from build123d import *

# Parameters (mm, degrees)
F1_DEPTH = 2
F2_DEPTH = 100
F4_DEPTH = 28.001


with BuildPart() as f1:
    # F0 (on Top) → F1 (new body)
    with BuildSketch(Plane.XY):
        with BuildLine():
            ThreePointArc((23.5, 0), (19.9852813742, 8.4852813742), (11.5, 12))
            Line((11.5, 12), (-4.2888974491, 12))
            ThreePointArc((-4.2888974491, 12), (0.6851433252, 6.8936407031), (2.5, 0))
            ThreePointArc((2.5, 0), (0.6851433252, -6.8936407031), (-4.2888974491, -12))
            Line((-4.2888974491, -12), (11.5, -12))
            ThreePointArc((11.5, -12), (19.9852813742, -8.4852813742), (23.5, 0))
        make_face()
        with BuildLine():
            ThreePointArc((2.5, 0), (0.6851433252, 6.8936407031), (-4.2888974491, 12))
            Line((-4.2888974491, 12), (-11.5, 12))
            ThreePointArc((-11.5, 12), (-19.9852813742, 8.4852813742), (-23.5, 0))
            ThreePointArc((-23.5, 0), (-19.9852813742, -8.4852813742), (-11.5, -12))
            Line((-11.5, -12), (-4.2888974491, -12))
            ThreePointArc((-4.2888974491, -12), (0.6851433252, -6.8936407031), (2.5, 0))
        make_face()
        with BuildLine():
            Line((-4.2888974491, 12), (11.5, 12))
            ThreePointArc((11.5, 12), (19.9852813742, 8.4852813742), (23.5, 0))
            ThreePointArc((23.5, 0), (19.9852813742, -8.4852813742), (11.5, -12))
            Line((11.5, -12), (-4.2888974491, -12))
            ThreePointArc((-4.2888974491, -12), (-7.7583426132, -13.4907375632), (-11.5, -14))
            Line((-11.5, -14), (11.5, -14))
            ThreePointArc((11.5, -14), (21.3994949366, -9.8994949366), (25.5, 0))
            ThreePointArc((25.5, 0), (21.3994949366, 9.8994949366), (11.5, 14))
            Line((11.5, 14), (-11.5, 14))
            ThreePointArc((-11.5, 14), (-7.7583426132, 13.4907375632), (-4.2888974491, 12))
        make_face()
        with BuildLine():
            Line((-11.5, 12), (-4.2888974491, 12))
            ThreePointArc((-4.2888974491, 12), (-7.7583426132, 13.4907375632), (-11.5, 14))
            ThreePointArc((-11.5, 14), (-25.5, 0), (-11.5, -14))
            ThreePointArc((-11.5, -14), (-7.7583426132, -13.4907375632), (-4.2888974491, -12))
            Line((-4.2888974491, -12), (-11.5, -12))
            ThreePointArc((-11.5, -12), (-19.9852813742, -8.4852813742), (-23.5, 0))
            ThreePointArc((-23.5, 0), (-19.9852813742, 8.4852813742), (-11.5, 12))
        make_face()
    extrude(amount=F1_DEPTH)

    # F0 (on Top) → F2 (join)
    with BuildSketch(Plane.XY):
        with BuildLine():
            Line((-4.2888974491, 12), (11.5, 12))
            ThreePointArc((11.5, 12), (19.9852813742, 8.4852813742), (23.5, 0))
            ThreePointArc((23.5, 0), (19.9852813742, -8.4852813742), (11.5, -12))
            Line((11.5, -12), (-4.2888974491, -12))
            ThreePointArc((-4.2888974491, -12), (-7.7583426132, -13.4907375632), (-11.5, -14))
            Line((-11.5, -14), (11.5, -14))
            ThreePointArc((11.5, -14), (21.3994949366, -9.8994949366), (25.5, 0))
            ThreePointArc((25.5, 0), (21.3994949366, 9.8994949366), (11.5, 14))
            Line((11.5, 14), (-11.5, 14))
            ThreePointArc((-11.5, 14), (-7.7583426132, 13.4907375632), (-4.2888974491, 12))
        make_face()
        with BuildLine():
            Line((-11.5, 12), (-4.2888974491, 12))
            ThreePointArc((-4.2888974491, 12), (-7.7583426132, 13.4907375632), (-11.5, 14))
            ThreePointArc((-11.5, 14), (-25.5, 0), (-11.5, -14))
            ThreePointArc((-11.5, -14), (-7.7583426132, -13.4907375632), (-4.2888974491, -12))
            Line((-4.2888974491, -12), (-11.5, -12))
            ThreePointArc((-11.5, -12), (-19.9852813742, -8.4852813742), (-23.5, 0))
            ThreePointArc((-23.5, 0), (-19.9852813742, 8.4852813742), (-11.5, 12))
        make_face()
    extrude(amount=F2_DEPTH)

    # F3 (on face) → F4 (cut, through all)
    with BuildSketch(Plane(origin=(0, 14, 0), x_dir=(-1, 0, 0), z_dir=(0, 1, 0))):
        Polygon((-30, 127.5684932653), (-30, 100), (30, 80), (30, 127.5684932653), align=None)
    extrude(amount=-F4_DEPTH, mode=Mode.SUBTRACT)


solid = f1.part
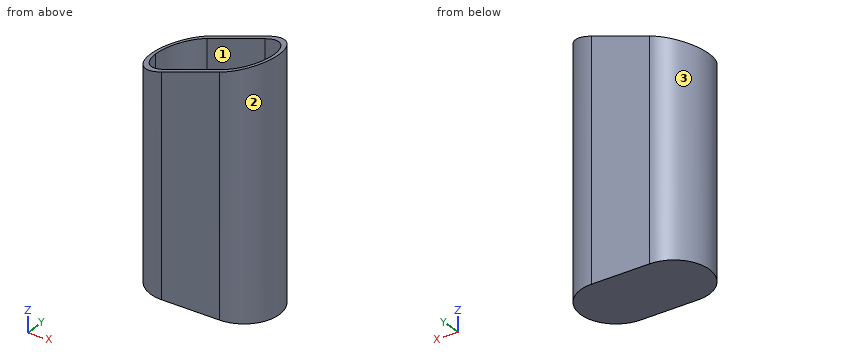
Input: part model. Units: mm. Frame: model coordinates. Face numbers are marked on the shaded views. Give positions to 0.01 mm unless a question says otherwise; leave off trailing zeros. Order: outer loops, then holes, each group sorted by start corner. A loop starts at its lowest first (then second) coordinate and runs counter-clockwise, first axis right, second up. Notation, with made-up numbers: (29, 78.5) - (76, 78.5) arc R11 ccw to (76, 94.5) - close; hole circle Ø9 at (14.5, 33.25). An arc over 180 degrees is marked (long way). Answer as a JSON object with one key per item and string values. Group by question number.
Q1. Cut plane C-C, the plane x = 20. Output: boundary loops of the cut face in (y, z), then the cut area to 3 significant figures.
Q2. Cut plane A-A, the plane z = 39. Output: boundary loops of the cut face in (x, y), then the cut area to 3 significant figures.
Q3. Mould query, pull axis X, two halves, no side actions, for the marked faces 1, 2 and 3. Classes: pulls with the +X half, pulls with the -X half, needs draft (parallel to the pull), parting line crosses it, or undercut.
Q4. Cut plane B-B, the plane y = 2.25. Output: boundary loops of the cut face in (x, z).
Q5. Line query: probe 1 along Y at (x, z) = (-11, 23); probe 2 along Y at (x, z) = (20, 53.5); probe 3 along Z at (x, y) = (-7, -6.75). Output: solid intervals per line, ascending.
Q6. First-contact query: pin 1 Ø7 at (x, y) = (9.5, -0.5) entering from +Z; pin 2 Ø2 at (y, z) = (-4, 24.5) entering from +X; pin 3 Ø1.5 at (x, z) = (-17, 27.5) entering from +Y. Flat tips, straight axial feed; report the tip coordinate or a pass-through.
Results:
{
 "1": {"outline": "(-11.12, 0) - (11.12, 0) - (11.12, 96.67) - (8.47, 96.67) - (8.47, 2) - (-8.47, 2) - (-8.47, 96.67) - (-11.12, 96.67) - close", "area": "547 mm^2"},
 "2": {"outline": "(-11.5, -14) - (11.5, -14) arc R14 ccw to (11.5, 14) - (-11.5, 14) arc R14 ccw to start; hole (-11.5, -12) - (11.5, -12) arc R12 ccw to (11.5, 12) - (-11.5, 12) arc R12 ccw to start", "area": "255 mm^2"},
 "3": {"face 1": "undercut", "face 2": "pulls with the +X half", "face 3": "pulls with the -X half"},
 "4": {"outline": "(-25.32, 0) - (25.32, 0) - (25.32, 98.44) - (23.29, 97.76) - (23.29, 2) - (-23.29, 2) - (-23.29, 82.24) - (-25.32, 81.56) - close"},
 "5": {"probe 1": "-14 to -12, 12 to 14", "probe 2": "-11.12 to -8.47, 8.47 to 11.12", "probe 3": "0 to 2"},
 "6": {"pin 1": "z = 2", "pin 2": "x = 25.17", "pin 3": "y = 13.17"}
}
